Check sheet for the modelled part. Datum: model origin and axes. Units: mm. A direction names the side the tool comes from. Coordinates: 2 decimals unless noted, no trailing zeros. Write each loop counter-clockwise with the first axis right and the second up, starting at its lowest first coordinate (ties: lowest second). Pieces come first, ordered by that corner, then holes. Notation, with made-up numbers: M 23.5,34.25 L 77.5,34.25 A15 cw 77.5,39.25 Z; hole C 81.5,31.5 d3. An arc over 180 degrees is marked long. Answer as CSV lines item,"result". Start each with the question number.
1) Section check A-A (x = -9). Record the cut outline in (y, z), and give its area (3 significant figures).
2) Section check B-B (z = 33). Record the cut outline in (x, y).
3) Go/stop test with flat-tipped pins: pin 1 Ø12 at (x, z) = (-2, -36) entering from +Y; pin 2 Ø3.5 at (x, z) = (48, 39.5) entering from -Y; pin 3 Ø7 at (x, y) = (32.5, 17.5) entering from -Z; pin 4 Ø3.5 at (y, z) = (1.5, 38.5) entering from +X. Record where each tip stops, or that it passes through.
4) Draft check along X on faces 5 (the flat face through (17.5, 1, -39)), 6 (the flat face through (-9, 0, -1)), 7 (the flat face through (47, 13, 0)). Enter one of: +X half, -X half, draft (parallel to the pull), parting line (faces both ways), or undercut.
5) Access from +Z, -Z, +X, -X, +Y, -Y to the whole of each face (thin tool, end or side, straight path). Record for faces 1 (the flat face through (14.5, 14, 48)), 2 (the flat face through (-23, 26, -1)), 3 (the flat face through (41, 2, -28.3)), 4 (the flat face through (0, 23, 46.6)).
6) Section check D-D (z = -16). Record the cut outline in (x, y), and give its area (3 significant figures).
7) Section check C-C (y = 20). Record the cut outline in (x, z), and give its area (3 significant figures).
8) Material ranges on L1, parallel to Y at x = 17, z = 44; L2, parallel to Z at x = -7, y = 12; L3, parallel to Y at x = 21.5, z = -39.5, recorded low to high. Write a range as [from, to].
Autodesk Inventor part; units mm, degrees
ref_plane "YZ Plane" through (0, 0, 0) normal (1, 0, 0) x (0, 1, 0)
ref_plane "XZ Plane" through (0, 0, 0) normal (0, 1, 0) x (-1, 0, 0)
ref_plane "XY Plane" through (0, 0, 0) normal (0, 0, 1) x (1, 0, 0)
sketch "Esboço1" plane through (0, 0, 0) normal (0, 1, 0) x (-1, 0, 0)
  line L0 (50, 50) -> (50, -50)
  line L1 (-50, -50) -> (-50, 50)
  line L2 (-50, -2) -> (-50, 2)
  line L3 (-50, -2) -> (-50, -28.3)
  line L4 (-50, 2) -> (-50, 28.3)
  line L5 (-50, 28.3) -> (-17.5, 28.3)
  line L6 (-50, -28.3) -> (-17.5, -28.3)
  line L7 (-17.5, -28.3) -> (-17.5, -49.6)
  line L8 (-17.5, 28.3) -> (-17.5, 49.6)
  line L9 (-39.9, -28.3) -> (-27.6, -28.3)
  line L10 (-27.6, -28.3) -> (-27.6, -2.3)
  line L11 (-27.6, -2.3) -> (-39.9, -2.3)
  line L12 (-39.9, -2.3) -> (-39.9, -28.3)
  line L13 (-27.6, 28.3) -> (-27.6, 2.3)
  line L14 (-27.6, 2.3) -> (-39.9, 2.3)
  line L15 (-39.9, 2.3) -> (-39.9, 28.3)
  line L16 (50, 50) -> (45, 50)
  line L17 (50, -50) -> (45, -50)
  line L18 (45, 50) -> (45, -50)
  line L19 (-17.5, -28.3) -> (-14.5, -28.3)
  line L20 (-14.5, -49.6) -> (-17.5, -49.6)
  line L21 (-17.5, 28.3) -> (-14.5, 28.3)
  line L22 (-14.5, 49.6) -> (-17.5, 49.6)
  line L23 (-9.5, -35) -> (-9.5, 35)
  line L24 (-9.5, -35) -> (24.5, -35)
  line L25 (24.5, -35) -> (24.5, 35)
  line L26 (24.5, 35) -> (-9.5, 35)
  line L27 (29.5, 35) -> (29.5, -35)
  line L28 (-14.5, 49.6) -> (29.5, 49.6)
  line L29 (29.5, 49.6) -> (29.5, -49.6)
  line L30 (29.5, -49.6) -> (-14.5, -49.6)
  line L31 (26.5, -46.6) -> (26.5, 46.6)
  line L32 (-14.5, -28.3) -> (-17.5, -28.3)
  line L33 (-14.5, -28.3) -> (-14.5, -46.6)
  line L34 (-14.5, 46.6) -> (-14.5, 28.3)
  line L35 (26.5, -46.6) -> (-14.5, -46.6)
  line L36 (26.5, 46.6) -> (-14.5, 46.6)
  line L37 (-50, 28.3) -> (-47, 28.3)
  line L38 (-47, 28.3) -> (-47, -28.3)
  line L39 (-14.5, -28.3) -> (-14.5, -25.3)
  line L40 (-14.5, -25.3) -> (-17.5, -25.3)
  line L41 (-17.5, -25.3) -> (-22.5, -25.3)
  line L42 (-22.5, -25.3) -> (-22.5, -28.3)
  line L43 (-14.5, 28.3) -> (-14.5, 25.3)
  line L44 (-14.5, 25.3) -> (-17.5, 25.3)
  line L45 (-17.5, 25.3) -> (-22.5, 25.3)
  line L46 (-22.5, 25.3) -> (-22.5, 28.3)
  point P0 (0, 0)
  point P1 (-50, 0)
  point P2 (-33.75, -28.3)
  dimension "d0" = 100
  dimension "d1" = 100
  dimension "d2" = 4
  dimension "d3" = 26.3
  dimension "d4" = 26.3
  dimension "d5" = 32.5
  dimension "d6" = 32.5
  dimension "d7" = 21.3
  dimension "d8" = 21.3
  dimension "d9" = 12.3
  dimension "d10" = 26
  dimension "d11" = 26
  dimension "d12" = 5
  dimension "d13" = 5
  dimension "d14" = 3
  dimension "d15" = 3
  dimension "d17" = 70
  dimension "d18" = 34
  dimension "d19" = 5
  dimension "d20" = 3
  dimension "d23" = 3
  dimension "d42" = 5
  dimension "d43" = 3
  dimension "d44" = 5
extrude "Extrusão1" add sketch "Esboço1" along normal blind 3 contours L38 L5 L15 L14 L13 L46 L45 L44 L43 L34 L36 L31 L35 L33 L39 L40 L41 L42 L6 L10 L11 L12 | L12 L11 L10 L6 | L5 L13 L14 L15 | L42 L41 L40 L39 L19 L6 | L5 L21 L43 L44 L45 L46 | L23 L26 L25 L24
extrude "Extrusão2" add sketch "Esboço1" along normal blind 27 contours L1 L5 L38 L6
sketch "Esboço2" plane through (14.5, 0, -46.6) normal (0, 0, -1) x (-1, 0, 0)
  line L0 (41, 0) -> (0, 0)
  line L1 (41, 0) -> (59.5, 0)
  line L2 (41, 0) -> (41, 3)
  line L3 (41, 0) -> (41, 3)
  line L4 (41, 3) -> (0, 3)
  line L5 (-32.5, 3) -> (0, 3)
  line L6 (-32.5, 3) -> (-32.5, 27)
  line L7 (-32.5, 27) -> (-32.5, 24)
  line L8 (-32.5, 27) -> (3, 27)
  line L9 (3, 27) -> (3, 24)
  line L10 (3, 24) -> (-32.5, 24)
  line L11 (0, 3) -> (0, 27)
  line L12 (0, 3) -> (3, 3)
  line L13 (3, 3) -> (37, 3)
  line L14 (0, 3) -> (-35.5, 3)
  line L15 (-35.5, 0) -> (-35.5, 27)
  line L16 (-11.75, 3) -> (-23.75, 3)
  line L17 (-23.75, 3) -> (-23.75, 15)
  line L18 (-23.75, 15) -> (-11.75, 15)
  line L19 (-11.75, 15) -> (-11.75, 3)
  line L20 (3, 3) -> (3, 21)
  line L21 (0, 27) -> (0, 42)
  line L22 (37, 3) -> (37, 21)
  line L23 (37, 21) -> (3, 21)
  line L24 (41, 3) -> (55.9231, 3)
  line L25 (0, 3) -> (41, 3)
  line L26 (-32.5, 27) -> (-35.5, 27)
  line L27 (-32.5, 27) -> (37.5, 27)
  line L28 (0, 42) -> (38, 42)
  line L29 (0, 42) -> (39.5, 42)
  line L30 (39.5, 42) -> (42.5, 32.2)
  line L31 (3, 24) -> (37.5, 24)
  line L32 (37.5, 24) -> (37.5, 27)
  line L33 (-23.75, 3) -> (-11.75, 15)
  line L34 (-23.75, 15) -> (-11.75, 3)
  line L35 (42.5, 3) -> (44, 3)
  line L36 (44, 3) -> (42.5, 32.2)
  line L37 (59.5, 0) -> (57, 0)
  line L38 (-17.75, 24) -> (-17.75, 3)
  line L39 (0, 27) -> (0, 37)
  line L40 (-35.5, 27) -> (-35.5, 32)
  line L41 (39.5, 42) -> (42.5, 42)
  line L42 (42.5, 32.2) -> (45.5, 32.2)
  line L43 (43.7518, 7.8322) -> (46.7478, 7.9861)
  line L44 (45.5, 32.2) -> (42.5, 42)
  line L45 (45.5, 32.2) -> (46.7478, 7.9861)
  line L46 (59.5, 0) -> (62, 0)
  line L47 (59.5, 0) -> (46.7478, 7.9861)
  line L48 (0, 42) -> (-35.5, 37.1)
  line L49 (-35.5, 37.1) -> (-35.5, 32)
  point P0 (14.5, 0)
  point P1 (0, 24)
  point P2 (54.7096, 3)
  dimension "d28" = 18.5
  dimension "d31" = 3
  dimension "d32" = 35.5
  dimension "d33" = 3
  dimension "d34" = 34
  dimension "d35" = 12
  dimension "d36" = 12
  dimension "d37" = 18
  dimension "d38" = 15
  dimension "d50" = 18
  dimension "d55" = 70
  dimension "d57" = 38
  dimension "d61" = 1.5
  dimension "d62" = 2.5
  dimension "d63" = 10
  dimension "d64" = 5
  dimension "d65" = 3
  dimension "d66" = 3
  dimension "d67" = 3
  dimension "d68" = 2.5
extrude "Extrusão3" add sketch "Esboço1" along normal blind 3 contours L19 L33 L35 L31 L36 L34 L21 L8 L22 L28 L29 L27 L30 L20 L7
extrude "Extrusão7" add sketch "Esboço2" along normal blind 3 contours L2 L24 L47 L1 | L4 L22 L23 L20 L11 L10 L31 L32 L27 L8 L21 L28 L29 L30 L36 L24 | L4 L20 L23 L22 | L11 L8 L9 L10 | L10 L6 L8 L11 | L9 L27 L32 L31 | L8 L26 L40 L49 L48 L21
mirror "Espelhar2" about plane through (0, 0, 0) normal (0, 0, 1) of "Extrusão7"
sketch "Esboço4" plane through (14.5, 0, -46.6) normal (0, 0, 1) x (1, 0, 0)
  line L0 (32.5, 27) -> (-37.5, 27)
  line L1 (-37.5, 27) -> (-37.5, 24)
  line L2 (-37.5, 24) -> (32.5, 24)
  line L3 (32.5, 24) -> (32.5, 27)
  line L4 (32.5, 27) -> (35.5, 27)
  line L5 (35.5, 27) -> (35.5, 24)
  line L6 (35.5, 24) -> (32.5, 24)
  point P0 (-14.5, 0)
  dimension "d71" = 70
  dimension "d72" = 3
  dimension "d73" = 3
  dimension "d74" = 3
extrude "Extrusão8" add sketch "Esboço4" along normal blind 96.2
sketch "Esboço5" plane through (14.5, 42, 46.6) normal (0, 0, -1) x (-1, 0, 0)
  line L0 (-32.5, -15) -> (-32.5, -18)
  line L1 (-32.5, -18) -> (-32.5117, -4.4875)
  line L2 (0, 0) -> (-35.5, -4.9)
  line L3 (-32.5117, -4.4875) -> (-35.5, -4.9)
  line L4 (-35.5, -18) -> (0, -18)
  line L5 (-35.5, -4.9) -> (-35.5, -18)
  line L6 (-35.5, -18) -> (-32.5, -18)
  point P0 (14.5, -42)
extrude "Extrusão9" add sketch "Esboço5" along normal blind 96.2
sketch "Esboço6" plane through (17.5, 0, -49.6) normal (0, 0, -1) x (-1, 0, 0)
  line L0 (42.5, 42) -> (3, 42)
  line L1 (42.5, 42) -> (45.5, 42)
  line L2 (47, 3) -> (45.5, 32.2)
  line L3 (45.5, 32.2) -> (48.5, 32.2)
  line L4 (46.7519, 7.8299) -> (49.7479, 7.9838)
  line L5 (57.7096, 3) -> (47, 3)
  line L6 (49.7479, 7.9838) -> (57.7096, 3)
  line L7 (49.7479, 7.9838) -> (48.5, 32.2)
  line L8 (45.5, 42) -> (48.5, 32.2)
  line L9 (45.5, 32.2) -> (42.5, 42)
  line L10 (42.5, 42) -> (45.5, 32.2)
  point P0 (17.5, 0)
  dimension "d79" = 3
  dimension "d80" = 3
  dimension "d81" = 3
sketch "Esboço7" plane through (14.5, 0, -46.6) normal (0, 0, 1) x (1, 0, 0)
  line L0 (-44, 3) -> (-44, 0)
  line L1 (-44, 3) -> (-44, 0)
  line L2 (-54.7096, 3) -> (-44, 3)
  line L3 (-44, 3) -> (-54.7096, 3)
  line L4 (-59.5, 0) -> (-54.7096, 3)
  line L5 (-54.7096, 3) -> (-59.5, 0)
  line L6 (-59.5, 0) -> (-44, 0)
  point P0 (-14.5, 0)
extrude "Extrusão10" add sketch "Esboço7" along normal blind 96.2
extrude "Extrusão11" add sketch "Esboço6" against normal blind 99.2
Results found:
1,outline,"M 0,-49.6 L 42,-49.6 L 42,-46.6 L 27,-46.6 L 27,46.6 L 42,46.6 L 42,49.6 L 0,49.6 Z; hole M 3,-46.6 L 24,-46.6 L 24,46.6 L 3,46.6 Z"
1,area,"811 mm2"
2,outline,"M -45,0 L 17.5,0 L 17.5,3 L -29.5,3 L -28,32.2 L -25,42 L -28,42 L -31,32.2 L -32.25,7.98 L -40.21,3 Z; M -23,24 L 50,24 L 50,37.1 L 47.01,37.51 L 47,27 L -23,27 Z"
3,pin 1,"stops at y = 27"
3,pin 2,"stops at y = 24"
3,pin 3,"passes through"
3,pin 4,"stops at x = 17.5"
4,face 5,"+X half"
4,face 6,"draft"
4,face 7,"undercut"
5,face 1,"+Z, -Z, +X"
5,face 2,"+Y"
5,face 3,"-Z, +X, -Y"
5,face 4,"none"
6,outline,"M -45,0 L 50,0 L 50,37.1 L 47.01,37.51 L 47,27 L -23,27 L -23,24 L 47,24 L 47,3 L -29.5,3 L -28,32.2 L -25,42 L -28,42 L -31,32.2 L -32.25,7.98 L -40.21,3 Z"
6,area,"727 mm2"
7,outline,"M -31.63,-49.6 L 14.5,-49.6 L 14.5,-46.6 L -28.63,-46.6 L -28.63,46.6 L 14.5,46.6 L 14.5,49.6 L -31.63,49.6 Z; M 47,-28.3 L 50,-28.3 L 50,28.3 L 47,28.3 Z"
7,area,"726 mm2"
8,L1,"y = [0, 3], [24, 27]"
8,L2,"z = [-49.6, -46.6], [46.6, 49.6]"
8,L3,"y = [24, 27]"
